from build123d import *

# Parameters (mm, degrees)
F1_DEPTH = 96.52
F0_R     = 45.239836
F2_DEPTH = 3.175
F4_D     = 32.766


with BuildPart() as f1:
    # F0 (on Top) → F1 (new body)
    with BuildSketch(Plane.XY):
        Polygon((27.57971, -4.723722), (17.880718, 21.522868), (-9.698991, 26.24659), (-27.57971, 4.723722), (-17.880718, -21.522868), (9.698991, -26.24659), align=None)
    extrude(amount=F1_DEPTH)

    # F0 (on Top) → F2 (join)
    with BuildSketch(Plane.XY):
        Circle(F0_R)
        Polygon((-9.698991, 26.24659), (17.880718, 21.522868), (27.57971, -4.723722), (9.698991, -26.24659), (-17.880718, -21.522868), (-27.57971, 4.723722), align=None, mode=Mode.SUBTRACT)
    extrude(amount=F2_DEPTH)

    # F4 (through all)
    with Locations(Plane(origin=(0, 0, 0), x_dir=(1, 0, 0), z_dir=(0, 0, -1))):
        with Locations((0, 0)):
            Hole(F4_D / 2)


solid = f1.part
Input: part model. Units: mm. Frame: model coordinates. A direction names the side the tool comes from. Round coordinates to 2 decimals unless told otherwise and drop trailing zeros. Order: outer loops, then holes, each group sorted by start corner. A loop starts at its lowest first (then second) coordinate and runs counter-clockwise, first axis right, second up. Notation, with made-up numbers: (36, 27.5) - (77, 27.5) arc R35 cw to (77, 60.5) - close; hole circle Ø5 at (38.25, 0.25). An arc over 180 degrees is marked (long way). Answer as a JSON object with one key per item and string values. Group by question number.
(1) Pin query (flat end, axial travel): P1, Ø2, axis at x = -12, y = 31.5, coming from the -Z side; P2, Ø2, axis at y = -3.5, z = 56, coming from the +X side; P3, Ø4, axis at x = -30, z = 55, coming from the -Y side; P4, Ø1, axis at y = -1, z = 35.5, coming from the -X side. Return the tip coordinate at first contact, or that it passes through.
(2) Cut plane C-C (y = 7). Return loops of the section in (x, z) (3 decimals).
(3) Material intervals for probe 1 along Z at (x, y) = (18, 23) (3 decimals); probe 2 along X at (y, z) = (10, 10.5); probe 3 along Y at (x, z) = (0, 69), sorted ascending. Write a range as from..to.
(4) Cut plane B-B (x = 0). Return loops of the section in (y, z) (3 decimals).
(5) Draft query along Y for faces 1 (the face through (19, -19, 3.175)), 2 (the face through (-15.626, -4.921, 48.936)), 3 (the face through (-4.284, -23.852, 49.194)). Return one class per face: released by +Y, released by -Y, zero draft, split by the parting line, or undercut.
(6) Cut plane A-A (z = 55). Return loops of the section in (x, y).
(7) Reachability of faces 4 (the face through (4.284, 23.852, 49.194)), 5 (the face through (18.51, -15.64, 49.19)), 6 (the face through (-18.51, 15.64, 49.19)) from +Z, -Z, +X, -X, +Y, -Y: full face, straight path, thin tool, end or side. Return the list, or none.
(8) Cut plane D-D (x = 36). Return loops of the section in (y, z) (3 decimals).
Here are the results:
{
 "1": {"P1": "stops at z = 0", "P2": "stops at x = 27.5", "P3": "passes through", "P4": "stops at x = -25.65"},
 "2": {"outline": "(-44.695, 0) - (-14.812, 0) - (-14.812, 96.52) - (-25.689, 96.52) - (-25.689, 3.175) - (-44.695, 3.175) - close; (14.812, 0) - (44.695, 0) - (44.695, 3.175) - (23.247, 3.175) - (23.247, 96.52) - (14.812, 96.52) - close"},
 "3": {"probe 1": "z = 0..3.175", "probe 2": "x = -23.2..-12.98, 12.98..22.14", "probe 3": "y = -24.59..-16.38, 16.38..24.59"},
 "4": {"outline": "(-45.24, 0) - (-16.383, 0) - (-16.383, 96.52) - (-24.585, 96.52) - (-24.585, 3.175) - (-45.24, 3.175) - close; (16.383, 0) - (45.24, 0) - (45.24, 3.175) - (24.585, 3.175) - (24.585, 96.52) - (16.383, 96.52) - close"},
 "5": {"face 1": "zero draft", "face 2": "undercut", "face 3": "released by -Y"},
 "6": {"outline": "(-27.58, 4.72) - (-17.88, -21.52) - (9.7, -26.25) - (27.58, -4.72) - (17.88, 21.52) - (-9.7, 26.25) - close; hole circle Ø32.77 at (0, 0)"},
 "7": {"face 4": "+Z, +X, +Y", "face 5": "+Z, +X, -Y", "face 6": "+Z, -X, +Y"},
 "8": {"outline": "(-27.398, 0) - (27.398, 0) - (27.398, 3.175) - (-27.398, 3.175) - close"}
}
